from build123d import *

# Parameters (mm, degrees)
F0_W      = 120
F0_H      = 80
F1_DEPTH  = 25
F3_DEPTH  = 120.001
F5_DEPTH  = 120.001
F7_DEPTH  = 5
F9_DEPTH  = 150
F11_DEPTH = 5
F13_DEPTH = 170
F14_W     = 3.3992808312
F14_H     = 11.5154450741
F14_H_2   = 11.5925325081
F15_DEPTH = 1
F16_W     = 3.3992808312
F16_H     = 68.1857028604
F17_DEPTH = 1
F18_W     = 3.3992808312
F18_H     = 10.4094055069
F18_H_2   = 12.2191561386
F19_DEPTH = 1
F20_W     = 5.3057130426
F20_H     = 2.1054418758
F20_W_2   = 5.30571118
F21_DEPTH = 25
F24_DEPTH = 25
F23_R     = 0.785
F25_DEPTH = 25
F26_W     = 10.8015254887
F26_H     = 6.9811940193
F27_DEPTH = 0.2
F28_W     = 5
F28_H     = 8.15
F29_DEPTH = 2.2
F30_W     = 5
F30_H     = 0.4
F31_DEPTH = 2.1


with BuildPart() as f1:
    # F0 (on Top) → F1 (new body)
    with BuildSketch(Plane.XY):
        Rectangle(F0_W, F0_H)
    extrude(amount=F1_DEPTH)

    # F2 (on face) → F3 (cut, through all)
    with BuildSketch(Plane.YZ.offset(60)):
        Polygon((-40, 0), (-28.1857028604, 25), (-40, 25), align=None)
    extrude(amount=-F3_DEPTH, mode=Mode.SUBTRACT)

    # F4 (on face) → F5 (cut, through all)
    with BuildSketch(Plane.YZ.offset(60)):
        Polygon((40, 0), (40, 25), (28.1857009977, 0), align=None)
    extrude(amount=-F5_DEPTH, mode=Mode.SUBTRACT)

    # F6 (on face) → F7 (cut)
    with BuildSketch(Plane.YZ.offset(60)):
        Polygon((35.0798550639, 14.5885804668), (-33.1058470208, 14.5885804668), (-34.9799869852, 10.6227500364), (33.205714804, 10.6227500364), align=None)
    extrude(amount=-F7_DEPTH, mode=Mode.SUBTRACT)

    # F8 (on face) → F9 (cut)
    with BuildSketch(Plane.YZ.offset(55)):
        Polygon((-33.1058470208, 14.5885804668), (-34.9799869852, 10.6227500364), (-29.9799869852, 10.6227500364), (-29.9799869852, 14.5885804668), align=None)
    extrude(amount=-F9_DEPTH, mode=Mode.SUBTRACT)

    # F10 (on face) → F11 (cut)
    with BuildSketch(Plane(origin=(-60, 0, 0), x_dir=(0, -1, 0), z_dir=(-1, 0, 0))):
        Polygon((29.9799869852, 10.6227500364), (29.9799869852, 14.5885804668), (-35.0798550639, 14.5885804668), (-33.205714804, 10.6227500364), align=None)
    extrude(amount=-F11_DEPTH, mode=Mode.SUBTRACT)

    # F12 (on face) → F13 (cut)
    with BuildSketch(Plane(origin=(-55, 0, 0), x_dir=(0, -1, 0), z_dir=(-1, 0, 0))):
        Polygon((-30.0832055509, 14.5885804668), (-35.0798550639, 14.5885804668), (-33.205714804, 10.6227500364), (-30.0832055509, 10.6227500364), align=None)
    extrude(amount=-F13_DEPTH, mode=Mode.SUBTRACT)

    # F14 (on face) → F15 (cut)
    with BuildSketch(Plane(origin=(0, -32.6977921499, 15.4520572908), x_dir=(1, 0, 0), z_dir=(0, -0.9041265419, 0.4272647847))):
        with Locations((-21.9536880031, 4.8026827457)):
            Rectangle(F14_W, F14_H)
        with Locations((-21.9536880031, -11.1376703717)):
            Rectangle(F14_W, F14_H_2)
    extrude(amount=-F15_DEPTH, mode=Mode.SUBTRACT)

    # F16 (on face) → F17 (cut)
    with BuildSketch(Plane.XY.offset(25)):
        with Locations((-21.9536880031, 5.9071485698)):
            Rectangle(F16_W, F16_H)
    extrude(amount=-F17_DEPTH, mode=Mode.SUBTRACT)

    # F18 (on face) → F19 (cut)
    with BuildSketch(Plane(origin=(0, 23.0402534943, -10.8881777548), x_dir=(-1, 0, 0), z_dir=(0, 0.9041265159, -0.4272648398))):
        with Locations((21.9536880031, 33.3830138355)):
            Rectangle(F18_W, F18_H)
        with Locations((21.9536880031, 17.6823684014)):
            Rectangle(F18_W, F18_H_2)
    extrude(amount=-F19_DEPTH, mode=Mode.SUBTRACT)

    # F20 (on face) → F21 (cut)
    with BuildSketch(Plane.XZ.offset(29.9799869852)):
        with Locations((21.8807244673, 12.5863919966)):
            Rectangle(F20_W, F20_H)
        with Locations((32.071063295, 12.5863919966)):
            Rectangle(F20_W_2, F20_H)
    extrude(amount=-F21_DEPTH, mode=Mode.SUBTRACT)

    # F22 (on face) → F24 (cut)
    with BuildSketch(Plane(origin=(0, 23.0402534943, -10.8881777548), x_dir=(-1, 0, 0), z_dir=(0, 0.9041265159, -0.4272648398))):
        with BuildLine():
            ThreePointArc((-44.3166374787, 16.9950310891), (-43.875457386, 17.751342396), (-43.7221280526, 18.6133962125))
            ThreePointArc((-43.7221280526, 18.6133962125), (-43.875457386, 19.4754500289), (-44.3166374787, 20.2317613358))
            ThreePointArc((-44.3166374787, 20.2317613358), (-44.9111469047, 18.6133962125), (-44.3166374787, 16.9950310891))
        make_face()
        with BuildLine():
            ThreePointArc((-44.3166374787, 16.9950310891), (-44.9111469047, 18.6133962125), (-44.3166374787, 20.2317613358))
            ThreePointArc((-44.3166374787, 20.2317613358), (-48.7221280526, 18.6133962125), (-44.3166374787, 16.9950310891))
        make_face()
        with BuildLine():
            ThreePointArc((-44.3166374787, 20.2317613358), (-43.875457386, 19.4754500289), (-43.7221280526, 18.6133962125))
            ThreePointArc((-43.7221280526, 18.6133962125), (-43.875457386, 17.751342396), (-44.3166374787, 16.9950310891))
            ThreePointArc((-44.3166374787, 16.9950310891), (-41.5490930882, 16.2667255459), (-39.9111469047, 18.6133962125))
            ThreePointArc((-39.9111469047, 18.6133962125), (-41.5490930882, 20.9600668791), (-44.3166374787, 20.2317613358))
        make_face()
    extrude(amount=-F24_DEPTH, mode=Mode.SUBTRACT)

    # F23 (on face) → F25 (join)
    with BuildSketch(Plane(origin=(0, 23.0402534943, -10.8881777548), x_dir=(-1, 0, 0), z_dir=(0, 0.9041265159, -0.4272648398))):
        with Locations((-42.3572132297, 18.6463277787)):
            Circle(F23_R)
        with Locations((-46.2783562048, 18.6463277787)):
            Circle(F23_R)
    extrude(amount=-F25_DEPTH)

    # F26 (on face) → F27 (cut)
    with BuildSketch(Plane(origin=(0, 23.0402534943, -10.8881777548), x_dir=(-1, 0, 0), z_dir=(0, 0.9041265159, -0.4272648398))):
        with Locations((-44.3166374787, 18.5013003647)):
            Rectangle(F26_W, F26_H)
        with BuildLine():
            ThreePointArc((-44.3166374787, 16.9950310891), (-48.7221280526, 18.6133962125), (-44.3166374787, 20.2317613358))
            ThreePointArc((-44.3166374787, 20.2317613358), (-39.9111469047, 18.6133962125), (-44.3166374787, 16.9950310891))
        make_face(mode=Mode.SUBTRACT)
    extrude(amount=-F27_DEPTH, mode=Mode.SUBTRACT)

    # F28 (on face) → F29 (cut)
    with BuildSketch(Plane(origin=(0, 23.0402534943, -10.8881777548), x_dir=(-1, 0, 0), z_dir=(0, 0.9041265159, -0.4272648398))):
        with Locations((50.181994272, 33.814091168)):
            Rectangle(F28_W, F28_H)
        with Locations((43.5504163067, 33.814091168)):
            Rectangle(F28_W, F28_H)
        with Locations((36.7609430726, 33.814091168)):
            Rectangle(F28_W, F28_H)
        with Locations((30.1819981592, 33.814091168)):
            Rectangle(F28_W, F28_H)
    extrude(amount=-F29_DEPTH, mode=Mode.SUBTRACT)

    # F30 (on face) → F31 (join)
    with BuildSketch(Plane(origin=(0, 23.0402534943, -10.8881777548), x_dir=(-1, 0, 0), z_dir=(0, 0.9041265159, -0.4272648398))):
        with Locations((50.181994272, 36.916055125)):
            Rectangle(F30_W, F30_H)
        with Locations((43.5504163067, 36.916055125)):
            Rectangle(F30_W, F30_H)
        with Locations((50.181994272, 35.3494960487)):
            Rectangle(F30_W, F30_H)
        with Locations((43.5504163067, 35.3494960487)):
            Rectangle(F30_W, F30_H)
        with Locations((43.5504163067, 33.614091168)):
            Rectangle(F30_W, F30_H)
        with Locations((50.181994272, 33.614091168)):
            Rectangle(F30_W, F30_H)
        with Locations((50.181994272, 31.5114263117)):
            Rectangle(F30_W, F30_H)
        with Locations((43.5504163067, 31.5114263117)):
            Rectangle(F30_W, F30_H)
        with Locations((43.5504163067, 29.939091168)):
            Rectangle(F30_W, F30_H)
        with Locations((50.181994272, 29.939091168)):
            Rectangle(F30_W, F30_H)
        with Locations((30.1819981592, 36.916055125)):
            Rectangle(F30_W, F30_H)
        with Locations((36.7609430726, 36.916055125)):
            Rectangle(F30_W, F30_H)
        with Locations((36.7609430726, 35.3494960487)):
            Rectangle(F30_W, F30_H)
        with Locations((30.1819981592, 35.3494960487)):
            Rectangle(F30_W, F30_H)
        with Locations((30.1819981592, 33.614091168)):
            Rectangle(F30_W, F30_H)
        with Locations((36.7609430726, 33.614091168)):
            Rectangle(F30_W, F30_H)
        with Locations((30.1819981592, 31.5114263117)):
            Rectangle(F30_W, F30_H)
        with Locations((36.7609430726, 31.5114263117)):
            Rectangle(F30_W, F30_H)
        with Locations((30.1819981592, 29.939091168)):
            Rectangle(F30_W, F30_H)
        with Locations((36.7609430726, 29.939091168)):
            Rectangle(F30_W, F30_H)
    extrude(amount=-F31_DEPTH)


solid = f1.part
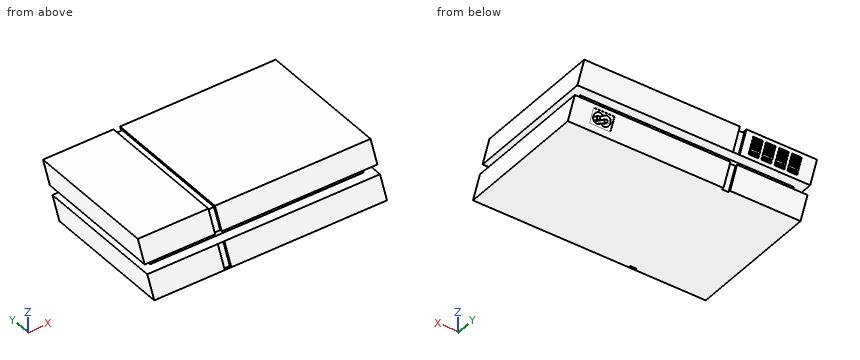
Geometry: final body of the model. Coordinates: model frame, mm. Give positions to 0.01 mm unless a question says otherwise; leave off trailing zeros. Write each loop counter-clockwise with the first axis right and the second up, starting at its lowest first coordinate (ties: lowest second). Pieces come first, ordered by that corner, then holes. Notation, with made-up numbers: (13.25, 30) -> (37.25, 30) arc R17 cw to (37.25, 57) -> close; hole circle Ø10 at (-4.5, -38.5). An arc over 180 degrees is marked (long way). Answer as a JSON object with one key per item and string values.
1. Cut plane A-A on y = -18.5. Output: boundary loops of the cut face in (x, z).
Ans:
{"outline": "(-60, 0) -> (60, 0) -> (60, 10.62) -> (55, 10.62) -> (55, 14.59) -> (60, 14.59) -> (60, 25) -> (-20.25, 25) -> (-20.25, 24) -> (-23.65, 24) -> (-23.65, 25) -> (-60, 25) -> (-60, 14.59) -> (-55, 14.59) -> (-55, 10.62) -> (-60, 10.62) -> close; hole (19.23, 11.53) -> (24.53, 11.53) -> (24.53, 13.64) -> (19.23, 13.64) -> close; hole (29.42, 11.53) -> (34.72, 11.53) -> (34.72, 13.64) -> (29.42, 13.64) -> close"}
2. Cut plane D-D on y = 25. Count the separate pieces of the cut face and the enclosed holes in it, and give its area (3 significant figures).
Ans:
{"separate pieces": "3", "enclosed holes": "1", "area": "2,920 mm^2"}
3. Cut plane C-C on x = 0. Output: boundary loops of the cut face in (y, z), and give its area (3 significant figures).
Ans:
{"outline": "(-40, 0) -> (28.19, 0) -> (33.21, 10.62) -> (30.08, 10.62) -> (30.08, 14.59) -> (35.08, 14.59) -> (40, 25) -> (-28.19, 25) -> (-33.11, 14.59) -> (-29.98, 14.59) -> (-29.98, 10.62) -> (-34.98, 10.62) -> close", "area": "1,670 mm^2"}
4. Ray query, probe 1 along Z at (x, y) = (34, -27.5); probe 2 along Y at (x, z) = (11, 13.75); probe 3 along X at (y, z) = (-20.5, 14). Return the intervals inside material, ascending. Write a range as from..to.
Ans:
{"probe 1": "z = 0..11.53, 13.64..25", "probe 2": "y = -29.98..30.08", "probe 3": "x = -55..55"}
5. Cut plane B-B on x = 32.5. Output: boundary loops of the cut face in (y, z).
Ans:
{"outline": "(-40, 0) -> (28.19, 0) -> (33.21, 10.62) -> (30.08, 10.62) -> (30.08, 14.59) -> (35.08, 14.59) -> (40, 25) -> (-28.19, 25) -> (-33.11, 14.59) -> (-29.98, 14.59) -> (-29.98, 13.64) -> (-4.98, 13.64) -> (-4.98, 11.53) -> (-29.98, 11.53) -> (-29.98, 10.62) -> (-34.98, 10.62) -> close"}
6. Contact query for flat-ended pins moving along their axis: pin 1 (4 mm diameter, centred on x = -21, z = 2.5, fed in from -Y); pin 2 (1.7 mm diameter, centred on y = -12, z = 12, fed in from +X); pin 3 (3 mm diameter, centred on x = 33, z = 17.5, fed in from -Y). Output: stop coordinate, or through.
Ans:
{"pin 1": "stops at y = -39.7", "pin 2": "stops at x = 55", "pin 3": "stops at y = -32.44"}
